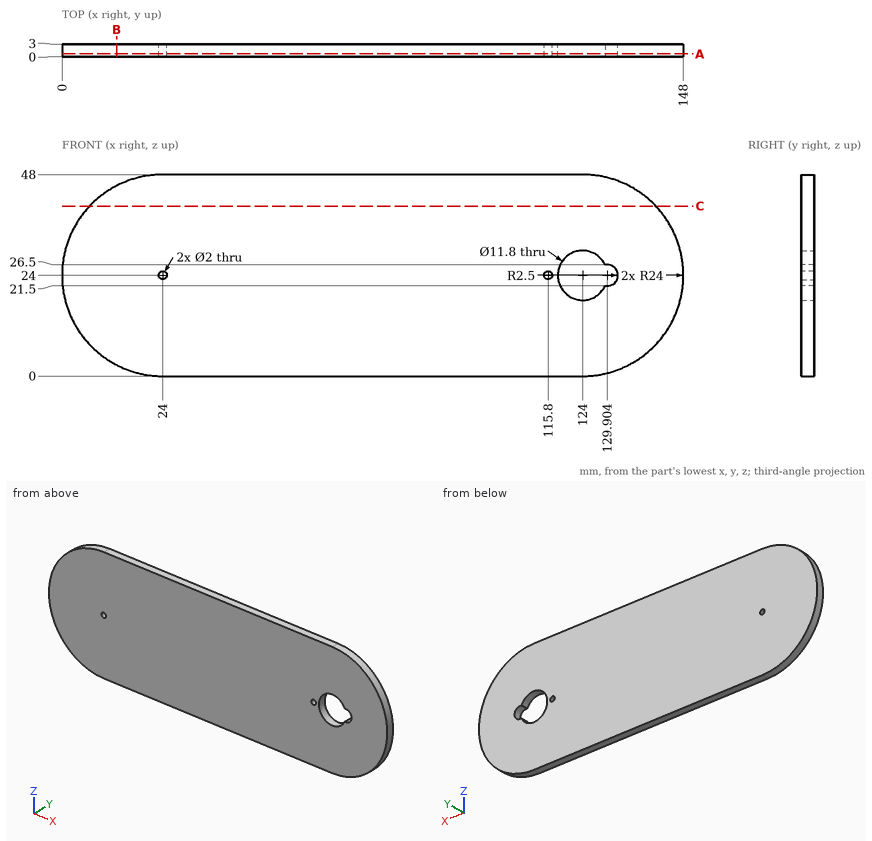
Design review of the part shown in the three views and the two pictorial views. Dimensions are in mm from the part's minimum x, y and z. Give positions to 0.01 mm unless a question says otherwise; leave off trailing zeros. Write each loop counter-clockwise with the first axis right and the second up, starting at its lowest first coordinate (ties: lowest second). Pieces come first, ordered by that corner, then holes. Notation, with made-up numbers: M 12.25,-37 L 28.25,-37 A35 ccw 28.25,0 Z; hole C 34,57.25 d11. An arc over 180 degrees is marked long. One line per question, with ' | ' between items. Start each with the question number.
Item 1: For pin 1 (1.5 mm diameter, centred on y = 2.5, z = 7.5, fed in from -X); pin 2 (12 mm diameter, centred on x = 77, z = 20, fed in from -Y); pin 3 (1.5 mm diameter, centred on x = 21.5, y = 0.5, fed in from -Z), all flat-tipped, find the tip position at first contact; note any pin that passes through.
Item 2: We need section C-C on z = 40.5. Write out the cut boundary in (x, y).
Item 3: Wall thickness on line 1 (X direction, y = 1.15, z = 24); line 2 (Z direction, x = 124, y = 1.1); line 3 (X direction, y = 2.15, z = 27): over which ranges is each line inside the solid? List them lowest first. Write a range as from..to.
Item 4: We need section A-A on y = 0.65. Write out the cut boundary in (x, z).
Item 5: We need section B-B on x = 13. Write out the cut boundary in (y, z), plus the area to 3 significant figures.
Results found:
1) pin 1: stops at x = 5.89 | pin 2: stops at y = 0 | pin 3: stops at z = 0.06
2) outline: M 6.57,0 L 141.43,0 L 141.43,3 L 6.57,3 Z
3) line 1: x = 0..23, 25..114.8, 116.8..118.1, 132.4..148 | line 2: z = 0..18.1, 29.9..48 | line 3: x = 0.19..118.92, 129.08..147.81
4) outline: M 24,0 L 124,0 A24 ccw 124,48 L 24,48 A24 ccw Z; hole C 24,24 d2; hole C 115.8,24 d2; hole M 129.34,21.5 L 129.9,21.5 A2.5 ccw 129.9,26.5 L 129.34,26.5 A5.9 ccw long Z
5) outline: M 0,2.67 L 3,2.67 L 3,45.33 L 0,45.33 Z | area: 128 mm2
